Geometry check sheet. Reference: the model listing, model coordinates, mm. A direction names the side the tool comes from. Give positions to 0.01 mm unless a question says otherwise; leave off trailing zeros. Loops run counter-clockwise (first coordinate to the right, second up) from the corner with the lowest first, then second, coordinate; pieces in that order, holes last. Notation, with made-up numbers: (-37, 15) -> (-5, 15) arc R31 ccw to (-5, 46) -> close; hole circle Ø6 at (74, 36.25). An arc over 180 degrees is marked (long way). Write item = value, one per line.
```python
from build123d import *

# Parameters (mm, degrees)
CROQUIS1_W              = 38.1
CROQUIS1_H              = 6.31
SALIENTE_EXTRUIR1_DEPTH = 340.39
CROQUIS3_W              = 38.1
CROQUIS3_H              = 6.31
SALIENTE_EXTRUIR2_DEPTH = 652.48
CROQUIS5_R              = 6.35
CORTAR_EXTRUIR1_DEPTH   = 6.31


with BuildPart() as part:
    # Croquis1 → Saliente-Extruir1 (new body)
    with BuildSketch(Plane.XY):
        Rectangle(CROQUIS1_W, CROQUIS1_H)
    extrude(amount=SALIENTE_EXTRUIR1_DEPTH)

    # Croquis3 → Saliente-Extruir2 (add)
    with BuildSketch(Plane.XZ.offset(3.155)):
        with Locations((0, 337.235)):
            Rectangle(CROQUIS3_W, CROQUIS3_H)
    extrude(amount=SALIENTE_EXTRUIR2_DEPTH)

    # Croquis5 → Cortar-Extruir1 (cut)
    with BuildSketch(Plane(origin=(0, 3.155, 0), x_dir=(1, 0, 0), z_dir=(0, 1, 0))):
        with Locations(Location((0, -43.892204666, 0), (0, 0, 270))):
            Circle(CROQUIS5_R)
        with Locations(Location((0, -11.892204666, 0), (0, 0, 270))):
            Circle(CROQUIS5_R)
    extrude(amount=-CORTAR_EXTRUIR1_DEPTH, mode=Mode.SUBTRACT)


solid = part.part
```
Item 1: Thickness scan on L1, parallel to Y at x = 5.5, z = 268 (3 decimals); L2, parallel to Z at x = 2.5, y = -354. Record the ranges inside material, lowest first. Write a range as [from, to].
Answer:
L1 = [-3.155, 3.155]
L2 = [334.08, 340.39]
Item 2: Tool access check on faces 5 (the flat face through (0, -3.155, 165)), 6 (the cylindrical face through (1.91, 0.04, 17.95)). Record the directions out of +Z, -Z, +X, -X, +Y, -Y that give a thin tool (end or side, any length) a straight path to the whole face; none if there is none.
Answer:
face_5 = -Z, +X, -X, -Y
face_6 = +Y, -Y
Item 3: Draft check along Z on faces 1 (the flat face through (0, 3.155, 168)), 2 (the flat face through (0, -325, 334.08)), 3 (the cylindrical face through (0.28, 0.04, 37.55)), 4 (the flat face through (0, -322, 340.39)). Enter one of: +Z half, -Z half, draft (parallel to the pull), parting line (faces both ways), or undercut.
Answer:
face_1 = draft
face_2 = -Z half
face_3 = undercut
face_4 = +Z half
Item 4: Section check B-B, the plane z = 284.5. Record the cut outline in (x, y) (3 decimals).
Answer:
outline = (-19.05, -3.155) -> (19.05, -3.155) -> (19.05, 3.155) -> (-19.05, 3.155) -> close
Item 5: Section check C-C, the plane y = -418. Record the cut outline in (x, z), plus the area to 3 significant figures.
Answer:
outline = (-19.05, 334.08) -> (19.05, 334.08) -> (19.05, 340.39) -> (-19.05, 340.39) -> close
area = 240 mm^2
Item 6: Gauge pin test, flat ends, axial feed: pin 1 (19 mm diameter, centred on x = -5.5, z = 211, fed in from -Y) (3 decimals); pin 2 (8 mm diameter, centred on x = 3, y = -369, fed in from -Z); pin 3 (11.5 mm diameter, centred on x = 0, z = 43.89, fed in from -Y); pin 4 (16.5 mm diameter, centred on x = 0, z = 11.89, fed in from +Y) (3 decimals). Record the tip position at first contact, or that the pin passes through.
Answer:
pin_1 = -3.155
pin_2 = 334.08
pin_3 = through
pin_4 = 3.155
Item 7: Section check A-A, the plane x = 0. Record the cut outline in (y, z) (3 decimals).
Answer:
outline = (-655.635, 334.08) -> (-3.155, 334.08) -> (-3.155, 50.242) -> (3.155, 50.242) -> (3.155, 340.39) -> (-655.635, 340.39) -> close; (-3.155, 0) -> (3.155, 0) -> (3.155, 5.542) -> (-3.155, 5.542) -> close; (-3.155, 18.242) -> (3.155, 18.242) -> (3.155, 37.542) -> (-3.155, 37.542) -> close
